Source: CAD feature listing. Evaluate the final solid. Frame: model axes, mm. Face numbers are marked on the shaded views. A direction names the side the tool comes from. Round coordinates to 2 decimals unless told otherwise and drop trailing zeros. Loops run counter-clockwise (first coordinate to the right, second up) from the corner with the lowest first, then second, coordinate; pieces in that order, holes last. Notation, with made-up numbers: M 63.25,-23 L 77.25,-23 A22 cw 77.25,7 Z; hole C 72.5,63 d3. An arc over 180 degrees is marked long. One line per item, written item: value.
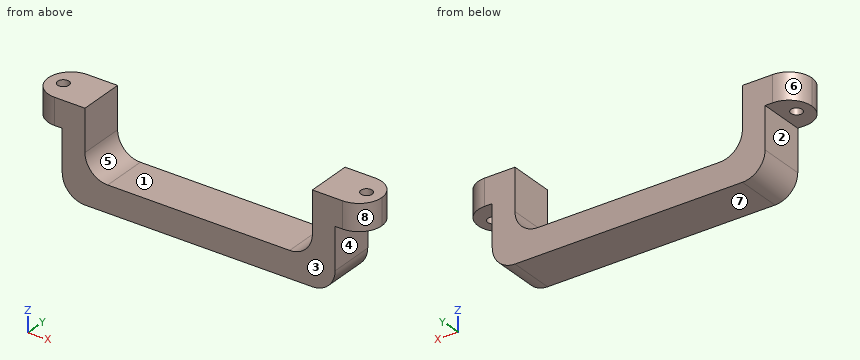
from build123d import *

# Parameters (mm, degrees)
EXTRUDE_2_DEPTH     = 12
SKETCH_6_R          = 1.5
CUT_EXTRUDE_2_DEPTH = 12
FILLET_2_R          = 6


with BuildPart() as part:
    # 草图3 → 凸台-拉伸2 (new body)
    with BuildSketch(Plane(origin=(0, 0, 0), x_dir=(1, 0, 0), z_dir=(0, 1, 0))):
        Polygon((0, 0), (14, 0), (14, 17), (74, 17), (74, 0), (88, 0), (88, 7), (80, 7), (80, 24), (8, 24), (8, 7), (0, 7), align=None)
    extrude(amount=EXTRUDE_2_DEPTH)

    # 草图6 → 切除-拉伸2 (cut)
    with BuildSketch(Plane(origin=(0, 0, -7), x_dir=(-1, 0, 0), z_dir=(0, 0, -1))):
        with Locations((-4, 6)):
            Circle(SKETCH_6_R)
        with Locations((-84, 6)):
            Circle(SKETCH_6_R)
    extrude(amount=-CUT_EXTRUDE_2_DEPTH, mode=Mode.SUBTRACT)

    # 圆角2
    fillet_2_edges = [part.edges().sort_by_distance(p)[0] for p in [
        (14, 6, -17),
        (8, 6, -24),
        (80, 6, -24),
        (74, 6, -17),
        (0, 12, -3.5),
        (0, 0, -3.5),
        (88, 12, -3.5),
        (88, 0, -3.5),
    ]]
    fillet(fillet_2_edges, radius=FILLET_2_R - 0.0001)  # a hair under: the kernel refuses the full size


solid = part.part
1. Reachability of the marked faces 1, 2, 3 and 4 from +Z, -Z, +X, -X, +Y, -Y: full face, straight path, thin tool, end or side. Return the list, or none.
Report:
face 1: +Z, +Y, -Y
face 2: -Z, -X, +Y, -Y
face 3: +Z, -Z, +X, -X, -Y
face 4: -Z, +X, +Y, -Y
2. Pin query (flat end, axial travel): pin 1 (6 mm diameter, centred on x = 36, y = 6.5, fed in from +Z); pin 2 (5.5 mm diameter, centred on y = 8.5, z = -14, fed in from +X); pin 3 (4 mm diameter, centred on x = 3.5, y = 4.5, fed in from -Z). Return the tip coordinate at first contact, or that it passes through.
Report:
pin 1: stops at z = -17
pin 2: stops at x = 80
pin 3: stops at z = -7
3. Section query D-D (y = 11.25). Return the cut outline in (x, z), and give its area (3 significant figures).
Report:
outline: M 3.1,-7 L 8,-7 L 8,-18 A6 ccw 14,-24 L 74,-24 A6 ccw 80,-18 L 80,-7 L 84.9,-7 L 84.9,0 L 74,0 L 74,-11 A6 cw 68,-17 L 20,-17 A6 cw 14,-11 L 14,0 L 3.1,0 Z
area: 777 mm2
4. Section query C-C (x = 4). Return the cut outline in (y, z).
Report:
outline: M 0.34,-7 L 4.5,-7 L 4.5,0 L 0.34,0 Z; M 7.5,-7 L 11.66,-7 L 11.66,0 L 7.5,0 Z
5. Section query B-B (z = -10). Return the cut outline in (x, y), and give its area (3 significant figures).
Report:
outline: M 8,0 L 14,0 L 14,12 L 8,12 Z; M 74,0 L 80,0 L 80,12 L 74,12 Z
area: 144 mm2
6. Pull-direction query (X, two-part tool) for the marked faces 5, 6, 7 and 8; classes: released by +X, released by -X, zero draft, split by the parting line, or undercut.
Report:
face 5: undercut
face 6: released by -X
face 7: zero draft
face 8: released by +X
7. Ray query, line 1 (X direction, y = 7, z = -5.5); line 2 (X direction, y = 4, z = -9.75); line 3 (Z direction, x = 82.5, y = 3.75). Return the intervals inside material, ascending. Write a range as [from, to].
Report:
line 1: x = [0.08, 2.88], [5.12, 14], [74, 82.88], [85.12, 87.92]
line 2: x = [8, 14], [74, 80]
line 3: z = [-7, 0]
8. Section query A-A (z = -6.25). Count the separate pieces of the cut face and the enclosed holes in it, and give its area (3 significant figures).
Report:
separate pieces: 2
enclosed holes: 2
area: 291 mm2
